```python
from build123d import *

# Parameters (mm, degrees)
F0_W     = 3.9
F0_H     = 3.5
F1_DEPTH = 0.7
F2_R     = 1.45
F3_DEPTH = 4
F5_DEPTH = 3
F6_SIZE  = 0.3
F8_DEPTH = 0.7


with BuildPart() as f1:
    # F0 (on Right) → F1 (new body)
    with BuildSketch(Plane.YZ):
        Rectangle(F0_W, F0_H)
        with BuildLine():
            Line((-1.95, 1.75), (1.95, 1.75))
            ThreePointArc((1.95, 1.75), (0, 3.7), (-1.95, 1.75))
        make_face()
        with BuildLine():
            ThreePointArc((-1.95, -1.75), (0, -3.7), (1.95, -1.75))
            Line((1.95, -1.75), (-1.95, -1.75))
        make_face()
    extrude(amount=F1_DEPTH)

    # F2 (on Right) → F3 (join)
    with BuildSketch(Plane.YZ):
        with Locations((0, 1.75)):
            Circle(F2_R)
    extrude(amount=F3_DEPTH)

    # F4 (on face) → F5 (join)
    with BuildSketch(Plane.YZ.offset(4)):
        Polygon((1.05, 1.143782), (1.05, 2.356218), (0, 2.962436), (-1.05, 2.356218), (-1.05, 1.143782), (0, 0.537564), align=None)
    extrude(amount=F5_DEPTH)

    # F6
    f6_edges = [f1.edges().sort_by_distance(p)[0] for p in [
        (7, -0.525, 2.659327),
        (7, 0.525, 2.659327),
        (7, 1.05, 1.75),
        (7, 0.525, 0.840673),
        (7, -0.525, 0.840673),
        (7, -1.05, 1.75),
    ]]
    chamfer(f6_edges, length=F6_SIZE)

    # F7 (on face) → F8 (cut, through all)
    with BuildSketch(Plane(origin=(0, 0, 0), x_dir=(0, -1, 0), z_dir=(-1, 0, 0))):
        Polygon((1.1, -2.385085), (1.1, -1.114915), (0, -0.479829), (-1.1, -1.114915), (-1.1, -2.385085), (0, -3.020171), align=None)
    extrude(amount=-F8_DEPTH, mode=Mode.SUBTRACT)


solid = f1.part
```
Read the model definition and answer for the solid it produces. Units are mm, in the model's axes. A direction names the side the tool comes from. Coordinates: 2 decimals unless noted, no trailing zeros. Order: outer loops, then holes, each group sorted by start corner. A loop starts at its lowest first (then second) coordinate and runs counter-clockwise, first axis right, second up. Notation, with made-up numbers: (-36, 5) - (8, 5) arc R18 cw to (8, 26) - close; hole circle Ø6 at (23.25, -3). An arc over 180 degrees is marked (long way). Answer as a JSON object with one key per item and string values. Group by question number.
Item 1: Section A-A (y = -0.2) is taken. Give the vertices of the cut face in (x, z), plus the area to 3 significant figures.
Item 2: Consider probe 1 along X at (y, z) = (-0.05, -3.5); probe 2 along Z at (x, y) = (3.5, -0.8); probe 3 along X at (y, z) = (-1.1, 2). Determine where each line is inside the solid, lowest interval first. Write a range as from..to.
Item 3: A tool of negligible diameter and unlimited length cuts with its end or side. For faces 1 (the face through (5, 1.05, 2)), 2 (the face through (5.33, -0.52, 2.66)), 3 (the face through (5, -1.05, 2)), 4 (the face through (5.33, 0.52, 0.84)), 5 (the face through (5.331, -0.532, 0.845)), from which of +Z, -Z, +X, -X, +Y, -Y can it reach the whole face along a straight path? Write none if from no direction.
Item 4: Section C-C (x = 2.75) is taken. Give the vertices of the cut face in (y, z).
Item 5: Section D-D (y = -0.9) is taken. Give the vertices of the cut face in (x, z), plus the area to 3 significant figures.
Item 6: Flat-ended cylindrical pins translate along their axes: P1, Ø1, axis at x = 6, z = 2, coming from the +Y side; P2, Ø2, axis at y = 0, z = -0.5, coming from the +X side; P3, Ø1.3, axis at x = 5, z = 1.5, coming from the -Y side; P4, Ø0.6, axis at x = 0.5, z = -2, coming from the +Y side. Find the tip coordinate at first contact, or state that the pin passes through.
Item 7: Section B-B (z = 1) is taken. Give the vertices of the cut face in (x, y).
Results are:
{
 "1": {"outline": "(0, -3.69) - (0.7, -3.69) - (0.7, -2.9) - (0, -2.9) - close; (0, -0.6) - (0.7, -0.6) - (0.7, 0.31) - (4, 0.31) - (4, 0.65) - (6.7, 0.65) - (7, 1) - (7, 2.5) - (6.7, 2.85) - (4, 2.85) - (4, 3.19) - (0.7, 3.19) - (0.7, 3.69) - (0, 3.69) - close", "area": "19.5 mm^2"},
 "2": {"probe 1": "x = 0..0.7", "probe 2": "z = 0.54..2.96", "probe 3": "x = 0..4"},
 "3": {"face 1": "+Z, -Z, +X, +Y", "face 2": "+Z, +X, -Y", "face 3": "+Z, -Z, +X, -Y", "face 4": "-Z, +X, +Y", "face 5": "-Z, +X, -Y"},
 "4": {"outline": "circle Ø2.9 at (0, 1.75)"},
 "5": {"outline": "(0, -3.48) - (0.7, -3.48) - (0.7, -2.5) - (0, -2.5) - close; (0, -1) - (0.7, -1) - (0.7, 0.61) - (4, 0.61) - (4, 1.06) - (6.7, 1.06) - (6.85, 1.23) - (6.85, 2.27) - (6.7, 2.44) - (4, 2.44) - (4, 2.89) - (0.7, 2.89) - (0.7, 3.48) - (0, 3.48) - close", "area": "15.2 mm^2"},
 "6": {"P1": "stops at y = 1.05", "P2": "stops at x = 4", "P3": "stops at y = -1.05", "P4": "stops at y = 1.95"},
 "7": {"outline": "(0, -1.95) - (0.7, -1.95) - (0.7, -1.24) - (4, -1.24) - (4, -0.8) - (6.7, -0.8) - (7, -0.2) - (7, 0.2) - (6.7, 0.8) - (4, 0.8) - (4, 1.24) - (0.7, 1.24) - (0.7, 1.95) - (0, 1.95) - close"}
}
